from build123d import *

# Parameters (mm, degrees)
F0_W     = 129.356236
F0_H     = 94.549194
F1_DEPTH = 25.4
F2_R     = 19.05
F3_DEPTH = 47.274597


with BuildPart() as f1:
    # F0 (on Top) → F1 (new body)
    with BuildSketch(Plane.XY):
        Rectangle(F0_W, F0_H)
    extrude(amount=F1_DEPTH)

    # F2 (on Front) → F3 (join, through all)
    with BuildSketch(Plane.XZ):
        with BuildLine():
            Line((-13.878118, 25.4), (-13.878118, 50.8))
            ThreePointArc((-13.878118, 50.8), (-39.278118, 76.2), (-64.678118, 50.8))
            Line((-64.678118, 50.8), (-64.678118, 25.4))
            Line((-64.678118, 25.4), (-13.878118, 25.4))
        make_face()
        with Locations((-39.278118, 50.8)):
            Circle(F2_R, mode=Mode.SUBTRACT)
    extrude(amount=F3_DEPTH)


solid = f1.part
The listing builds one solid part. Answer for the finished solid, in the listing's coordinates (mm). A direction names the side the tool comes from. Coordinates: 2 decimals unless noted, no trailing zeros. Write each loop counter-clockwise with the first axis right and the second up, starting at its lowest first coordinate (ties: lowest second). Pieces come first, ordered by that corner, then holes. Notation, with made-up numbers: M -26.75,-22.5 L 14.25,-22.5 A20 cw 14.25,-8.5 Z; hole C 27.5,33.25 d1. An arc over 180 degrees is marked long. Use one line per item in the form item = value.
Item 1: Given P1, Ø12.5, axis at y = -35.5, z = 41.5, coming from the +X side; P2, Ø10, axis at x = -28.5, y = -22, coming from the +Z side; P3, Ø23, axis at x = -39.28, z = 50.8, coming from the +Y side, each flat-ended and moving along its own axis, determine where each tip first touches the part or whether it passes through.
Model answer:
P1 = -13.88
P2 = 75.53
P3 = through
Item 2: Find the intervals of material crossed by probe 1 along X at (y, z) = (-35, 50); probe 2 along Z at (x, y) = (-39, 34.5); probe 3 along Y at (x, z) = (-25.5, 31.5), in increasing order.
Model answer:
probe_1 = -64.68 to -58.31, -20.24 to -13.88
probe_2 = 0 to 25.4
probe_3 = -47.27 to 0
Item 3: Find section C-C, the plane y = 9. Give the vertices of the cut face in (x, z), plus the area to 3 significant figures.
Model answer:
outline = M -64.68,0 L 64.68,0 L 64.68,25.4 L -64.68,25.4 Z
area = 3,290 mm2
Item 4: For faces 1 (the face through (-13.878, -23, 38)), 2 (the face through (13, 11, 25.4)), 3 (the face through (-28, 0, 34)), determine the directions among +Z, -Z, +X, -X, +Y, -Y from which every point of the face is accessible in a straight line to the end or side of a thin tool.
Model answer:
face_1 = +Z, +X, +Y, -Y
face_2 = +Z, +X, +Y
face_3 = +Z, +X, -X, +Y
Item 5: The mould has two halves that part along X. Classify faces 4 (the face through (64.678, -1, 13)), 5 (the face through (-43.4, -23.3, 32.2)), 6 (the face through (-1, 47.275, 13)), 7 (the face through (-64.678, -11, 19)): released by +X, released by -X, zero draft, split by the parting line, or undercut.
Model answer:
face_4 = released by +X
face_5 = undercut
face_6 = zero draft
face_7 = released by -X
Item 6: Find section A-A, the plane y = -4. Give the vertices of the cut face in (x, z).
Model answer:
outline = M -64.68,0 L 64.68,0 L 64.68,25.4 L -13.88,25.4 L -13.88,50.8 A25.4 ccw -64.68,50.8 Z; hole C -39.28,50.8 d38.1
Item 7: Find section B-B, the plane z = 61.5. Give the vertices of the cut face in (x, y).
Model answer:
outline = M -62.31,-47.27 L -55.04,-47.27 L -55.04,0 L -62.31,0 Z; M -23.52,-47.27 L -16.24,-47.27 L -16.24,0 L -23.52,0 Z
Item 8: Find section D-D, the plane x = 24. Give the vertices of the cut face in (y, z).
Model answer:
outline = M -47.27,0 L 47.27,0 L 47.27,25.4 L -47.27,25.4 Z
